from build123d import *

# Parameters (mm, degrees)
SKETCH3_R                = 16
SKETCH3_R_2              = 10
BOSS_EXTRUDE4_DEPTH      = 14
BOSS_EXTRUDE5_DEPTH      = 6
BOSS_EXTRUDE6_DEPTH      = 6
BOSS_EXTRUDE6_DEPTH_BACK = 24
SKETCH3_4_R              = 9
SKETCH3_4_R_2            = 3


with BuildPart() as part:
    # Sketch3 → Boss-Extrude4 (new body)
    with BuildSketch(Plane.XY):
        Circle(SKETCH3_R)
        Circle(SKETCH3_R_2, mode=Mode.SUBTRACT)
    extrude(amount=BOSS_EXTRUDE4_DEPTH)

    # Sketch3_3 → Boss-Extrude5 (add)
    with BuildSketch(Plane.XY):
        with BuildLine():
            ThreePointArc((58.430427234, -8.932663764), (48.331555959, 0), (58.430427234, 8.932663764))
            Line((58.430427234, 8.932663764), (1.953548933, 15.880291136))
            ThreePointArc((1.953548933, 15.880291136), (11.984506309, 10.600547558), (16, 0))
            ThreePointArc((16, 0), (11.984506309, -10.600547558), (1.953548933, -15.880291136))
            Line((1.953548933, -15.880291136), (58.430427234, -8.932663764))
        make_face()
    extrude(amount=BOSS_EXTRUDE5_DEPTH)

    # Sketch3_4 → Boss-Extrude6 (add, two sides: drawn at the far end of the back side and taken through both)
    with BuildSketch(Plane.XY.offset(-BOSS_EXTRUDE6_DEPTH_BACK)):
        with Locations((57.331555959, 0)):
            Circle(SKETCH3_4_R)
        with Locations((57.331555959, 0)):
            Circle(SKETCH3_4_R_2, mode=Mode.SUBTRACT)
    extrude(amount=BOSS_EXTRUDE6_DEPTH + BOSS_EXTRUDE6_DEPTH_BACK)


solid = part.part
Could you check a few things on this model? Use its own coordinates, in mm. A direction names the side the tool comes from. Give positions to 0.01 mm unless a question says otherwise; leave off trailing zeros. Order: outer loops, then holes, each group sorted by start corner. A loop starts at its lowest first (then second) coordinate and runs counter-clockwise, first axis right, second up.
Item 1: I need wall thicknesses on line 1 (Y direction, x = 0, z = 7.75); line 2 (Y direction, x = -5.5, z = 6); line 3 (Z direction, x = 24, y = -5). Which ranges of each line are inside material? Lowest first, please.
Item 2: I'm going to push flat-ended pins straight in: pin 1 (5 mm diameter, centred on x = 57.5, z = -18, fed in from -Y); pin 2 (12 mm diameter, centred on x = 0, y = 0, fed in from -Z); pin 3 (2 mm diameter, centred on x = 25, y = -3.5, fed in from -Z); pin 4 (16 mm diameter, centred on x = 30, y = -7.5, fed in from +Z). Where does each tip first touch, or does it pass through?
Item 3: For faces 1 (the face through (65.916, 2.703, -9.21)), 2 (the face through (-15.985, 0.703, 8.458)), 3 (the face through (29.797, -12.455, 2.958)), which set-ups out of +Z, -Z, +X, -X, +Y, -Y let a thin tool reach every point of the face, with its end or its side?
Item 4: If we mould it in two halves opening along X, with no side actions, what happens to faces 4 (the face through (10.4, 0.2, 14)), 5 (the face through (30.587, 12.358, 2.958)), 6 (the face through (-2.17, -9.76, 6.9))? For each: pulls with the +X half, pulls with the -X half, needs draft (parallel to the pull), parting line crosses it, or undercut.
Item 5: If we section it at B-B, the plane z = 2.5: Write out the boundary of the cut face in (x, y).
Item 6: If we section it at C-C, the plane x = 0: Write out the boundary of the cut face in (y, z), plus the area to 3 significant figures.
Item 7: If we section it at D-D, the plane y = 5: Write out the boundary of the cut face in (x, z).
Item 8: If we section it at A-A, the plane y = 0: Write out the boundary of the cut face in (x, z), plus the area to 3 significant figures.
Values:
1. line 1: y = -16 to -10, 10 to 16
1. line 2: y = -15.02 to -8.35, 8.35 to 15.02
1. line 3: z = 0 to 6
2. pin 1: stops at y = -9
2. pin 2: passes through
2. pin 3: stops at z = 0
2. pin 4: stops at z = 6
3. face 1: -Z
3. face 2: +Z
3. face 3: +Z, -Z, +X, -Y
4. face 4: needs draft
4. face 5: pulls with the +X half
4. face 6: undercut
5. outline: (1.95, -15.88) - (58.43, -8.93) arc R9 ccw to (58.43, 8.93) - (1.95, 15.88) arc R16 ccw (long way) to start; hole circle Ø20 at (0, 0); hole circle Ø6 at (57.33, 0)
6. outline: (-16, 0) - (-10, 0) - (-10, 14) - (-16, 14) - close; (10, 0) - (16, 0) - (16, 14) - (10, 14) - close
6. area: 168 mm2
7. outline: (-15.2, 0) - (-8.66, 0) - (-8.66, 14) - (-15.2, 14) - close; (8.66, 0) - (49.85, 0) - (49.85, -24) - (64.81, -24) - (64.81, 6) - (15.2, 6) - (15.2, 14) - (8.66, 14) - close
8. outline: (-16, 0) - (-10, 0) - (-10, 14) - (-16, 14) - close; (10, 0) - (48.33, 0) - (48.33, -24) - (54.33, -24) - (54.33, 6) - (16, 6) - (16, 14) - (10, 14) - close; (60.33, -24) - (66.33, -24) - (66.33, 6) - (60.33, 6) - close
8. area: 722 mm2
